Could you check a few things on this model? Use its own coordinates, in mm. Face numbers are marked on the shaded views. A direction names the side the tool comes from. Coordinates: 2 decimals unless noted, no trailing zeros. Loops run counter-clockwise (first coordinate to the right, second up) from the corner with the lowest first, then second, coordinate; pieces in that order, holes last. Notation, with made-up numbers: M 13,-21.75 L 52,-21.75 A17 cw 52,4.25 Z; hole C -32,65.5 d9. An arc over 180 degrees is marked long. Write each question's results on one line, items separated by ' | '.
```python
from build123d import *

# Parameters (mm, degrees)
BOSS_EXTRUDE1_DEPTH               = 25.4
BOSS_EXTRUDE1_DEPTH_BACK          = 25.4
SKETCH1_R                         = 4.445
SKETCH9_W                         = 30.48
SKETCH9_H                         = 35.052
CUT_EXTRUDE6_DEPTH                = 75.08914513
BOSS_EXTRUDE3_DEPTH               = 12.7
SKETCH11_W                        = 5.350768363
SKETCH11_H                        = 57.15
CUT_EXTRUDE7_DEPTH                = 94.35417198
SKETCH12_W                        = 30.48
SKETCH12_H                        = 19.05
CUT_EXTRUDE8_DEPTH                = 93.670395825
SKETCH14_R                        = 1.6
CUT_EXTRUDE9_DEPTH                = 81.005571081
SKETCH15_R                        = 3.429
CUT_EXTRUDE10_DEPTH               = 81.005571081
CUT_EXTRUDE11_DEPTH               = 2.778125
SKETCH22_W                        = 1.89865
SKETCH22_H                        = 38.369875
SKETCH23_R                        = 3.175
CUT_EXTRUDE12_DEPTH               = 22.225
SKETCH24_W                        = 43.18
SKETCH24_H                        = 41.402
CUT_EXTRUDE13_DEPTH               = 94.35417198
CUT_EXTRUDE14_REACH               = 74.389
SKETCH25_W                        = 12.7
SKETCH25_H                        = 19.05
CUT_EXTRUDE15_DEPTH               = 74.112136493
CUT_EXTRUDE15_DEPTH_BACK          = 74.112136493
SKETCH26_W                        = 19.05
SKETCH26_H                        = 61.020370042
F_25_0_1495_DIAMETER_HOLE1_REACH  = 58.443
F_25_0_1495_DIAMETER_HOLE1_BORE_R = 1.89865


with BuildPart() as part:
    # Sketch1 → Boss-Extrude1 (new, two sides: drawn at the far end of the back side and taken through both)
    with BuildSketch(Plane.XY.offset(-BOSS_EXTRUDE1_DEPTH_BACK)):
        with BuildLine():
            Line((-26.940768363, -17.415768363), (-26.940768363, 39.734231637))
            Line((-26.940768363, 39.734231637), (26.940768363, 39.734231637))
            Line((26.940768363, 39.734231637), (26.940768363, -17.415768363))
            ThreePointArc((26.940768363, -17.415768363), (36.465768363, -26.940768363), (26.940768363, -36.465768363))
            Line((26.940768363, -36.465768363), (-26.940768363, -36.465768363))
            ThreePointArc((-26.940768363, -36.465768363), (-36.465768363, -26.940768363), (-26.940768363, -17.415768363))
        make_face()
        with Locations((-26.940768363, -26.940768363)):
            Circle(SKETCH1_R, mode=Mode.SUBTRACT)
        with Locations((26.940768363, -26.940768363)):
            Circle(SKETCH1_R, mode=Mode.SUBTRACT)
    extrude(amount=BOSS_EXTRUDE1_DEPTH + BOSS_EXTRUDE1_DEPTH_BACK)

    # Sketch9 → Cut-Extrude6 (cut, through all)
    with BuildSketch(Plane.XY.offset(25.4)):
        with Locations((0, 22.208231637)):
            Rectangle(SKETCH9_W, SKETCH9_H)
    extrude(amount=-CUT_EXTRUDE6_DEPTH, mode=Mode.SUBTRACT)

    # Sketch10 → Boss-Extrude3 (add)
    with BuildSketch(Plane.XY.offset(25.4)):
        Polygon((-26.940768363, 39.734231637), (-26.940768363, -1.667768363), (26.940768363, -1.667768363), (26.940768363, 39.734231637), (15.24, 39.734231637), (15.24, 4.682231637), (-15.24, 4.682231637), (-15.24, 39.734231637), align=None)
    boss_extrude3 = extrude(amount=BOSS_EXTRUDE3_DEPTH)

    # Mirror4: Boss-Extrude3 across plane
    add(boss_extrude3.mirror(Plane.XY))

    # Sketch11 → Cut-Extrude7 (cut, through all)
    with BuildSketch(Plane.XY.offset(38.1)):
        with Locations((-24.265384181, 11.159231637)):
            Rectangle(SKETCH11_W, SKETCH11_H)
    cut_extrude7 = extrude(amount=-CUT_EXTRUDE7_DEPTH, mode=Mode.SUBTRACT)

    # Mirror5: Cut-Extrude7 across plane
    add(cut_extrude7.mirror(Plane(origin=(0, 0, 0), x_dir=(0, 0, 1), z_dir=(1, 0, 0))), mode=Mode.SUBTRACT)

    # Sketch12 → Cut-Extrude8 (cut, through all)
    with BuildSketch(Plane.XZ.offset(36.465768363)):
        Rectangle(SKETCH12_W, SKETCH12_H)
    extrude(amount=-CUT_EXTRUDE8_DEPTH, mode=Mode.SUBTRACT)

    # Sketch14 → Cut-Extrude9 (cut, through all)
    with BuildSketch(Plane.ZY.offset(21.59)):
        with Locations(Location((-18.4, 22.462231637, 0), (0, 0, 90))):
            Circle(SKETCH14_R)
    cut_extrude9 = extrude(amount=-CUT_EXTRUDE9_DEPTH, mode=Mode.SUBTRACT)

    # Mirror6: Cut-Extrude9 across plane
    add(cut_extrude9.mirror(Plane.XY), mode=Mode.SUBTRACT)

    # Sketch15 → Cut-Extrude10 (cut, through all)
    with BuildSketch(Plane(origin=(21.59, 0, 0), x_dir=(0, 0, -1), z_dir=(1, 0, 0))):
        with Locations(Location((0, 22.462231637, 0), (0, 0, 90))):
            Circle(SKETCH15_R)
    extrude(amount=-CUT_EXTRUDE10_DEPTH, mode=Mode.SUBTRACT)

    # Sketch18 → Cut-Extrude11 (cut)
    with BuildSketch(Plane(origin=(0, 4.682231637, 0), x_dir=(1, 0, 0), z_dir=(0, 1, 0))):
        Polygon((-15.24, 2.346351494), (-19.304, 4.692702988), (-23.368, 2.346351494), (-23.368, -2.346351494), (-19.304, -4.692702988), (-15.24, -2.346351494), align=None)
    cut_extrude11 = extrude(amount=-CUT_EXTRUDE11_DEPTH, mode=Mode.SUBTRACT)

    # Mirror7: Cut-Extrude11 across plane
    add(cut_extrude11.mirror(Plane(origin=(0, 0, 0), x_dir=(0, 0, 1), z_dir=(1, 0, 0))), mode=Mode.SUBTRACT)

    # Sketch22 → #6 Clearance Hole1 (revolve, cut)
    with BuildSketch(Plane(origin=(0, 1.904106637, -19.05), x_dir=(0, 0, 1), z_dir=(1, 0, 0))):
        with Locations((0.949325, 19.1849375)):
            Rectangle(SKETCH22_W, SKETCH22_H)
    f_6_clearance_hole1 = revolve(axis=Axis((0, 8.254106637, -19.05), (0, -1, 0)), mode=Mode.SUBTRACT)

    # Mirror8: #6 Clearance Hole1 across plane
    add(f_6_clearance_hole1.mirror(Plane.XY), mode=Mode.SUBTRACT)

    # Sketch23 → Cut-Extrude12 (cut)
    with BuildSketch(Plane.XZ.offset(36.465768363)):
        with Locations(Location((0, -19.05, 0), (0, 0, 270))):
            Circle(SKETCH23_R)
        with Locations(Location((0, 19.05, 0), (0, 0, 270))):
            Circle(SKETCH23_R)
    extrude(amount=-CUT_EXTRUDE12_DEPTH, mode=Mode.SUBTRACT)

    # Sketch24 → Cut-Extrude13 (cut, through all)
    with BuildSketch(Plane(origin=(0, 0, -38.1), x_dir=(-1, 0, 0), z_dir=(0, 0, -1))):
        with Locations((0, 19.033231637)):
            Rectangle(SKETCH24_W, SKETCH24_H)
    extrude(amount=-CUT_EXTRUDE13_DEPTH, mode=Mode.SUBTRACT)

    # Sketch25 → Cut-Extrude14 (cut, up to next)
    with BuildSketch(Plane.XY.offset(25.4), mode=Mode.PRIVATE) as cut_extrude14_sk1:
        with Locations((0, -19.05)):
            Rectangle(SKETCH25_W, SKETCH25_H)
    cut_extrude14_tool1 = extrude(cut_extrude14_sk1.sketch, amount=-CUT_EXTRUDE14_REACH, mode=Mode.PRIVATE) & part.part
    add(cut_extrude14_tool1.solids().sort_by_distance((0, -19.05, 25.4))[0], mode=Mode.SUBTRACT)

    # Sketch26 → Cut-Extrude15 (cut, two sides: drawn at the far end of the back side and taken through both)
    with BuildSketch(Plane(origin=(21.59, 0, 0), x_dir=(0, 0, -1), z_dir=(1, 0, 0)).offset(-CUT_EXTRUDE15_DEPTH_BACK)):
        with Locations((0, -47.925953384)):
            Rectangle(SKETCH26_W, SKETCH26_H)
    extrude(amount=CUT_EXTRUDE15_DEPTH + CUT_EXTRUDE15_DEPTH_BACK, mode=Mode.SUBTRACT)

    # #25 (0.1495) Diameter Hole1 bore → #25 (0.1495) Diameter Hole1 (cut, up to next)
    with BuildSketch(Plane(origin=(0, -36.465768363, 0), x_dir=(-1, 0, 0), z_dir=(0, -1, 0)), mode=Mode.PRIVATE) as f_25_0_1495_diameter_hole1_sk1:
        with Locations((26.940768363, -17.4625)):
            Circle(F_25_0_1495_DIAMETER_HOLE1_BORE_R)
    f_25_0_1495_diameter_hole1_tool1 = extrude(f_25_0_1495_diameter_hole1_sk1.sketch, amount=-F_25_0_1495_DIAMETER_HOLE1_REACH, mode=Mode.PRIVATE) & part.part
    # #25 (0.1495) Diameter Hole1 bore → #25 (0.1495) Diameter Hole1 (cut, up to next)
    with BuildSketch(Plane(origin=(0, -36.465768363, 0), x_dir=(-1, 0, 0), z_dir=(0, -1, 0)), mode=Mode.PRIVATE) as f_25_0_1495_diameter_hole1_sk2:
        with Locations((26.940768363, 17.4625)):
            Circle(F_25_0_1495_DIAMETER_HOLE1_BORE_R)
    f_25_0_1495_diameter_hole1_tool2 = extrude(f_25_0_1495_diameter_hole1_sk2.sketch, amount=-F_25_0_1495_DIAMETER_HOLE1_REACH, mode=Mode.PRIVATE) & part.part
    # #25 (0.1495) Diameter Hole1 bore → #25 (0.1495) Diameter Hole1 (cut, up to next)
    with BuildSketch(Plane(origin=(0, -36.465768363, 0), x_dir=(-1, 0, 0), z_dir=(0, -1, 0)), mode=Mode.PRIVATE) as f_25_0_1495_diameter_hole1_sk3:
        with Locations((-26.940768363, 17.4625)):
            Circle(F_25_0_1495_DIAMETER_HOLE1_BORE_R)
    f_25_0_1495_diameter_hole1_tool3 = extrude(f_25_0_1495_diameter_hole1_sk3.sketch, amount=-F_25_0_1495_DIAMETER_HOLE1_REACH, mode=Mode.PRIVATE) & part.part
    # #25 (0.1495) Diameter Hole1 bore → #25 (0.1495) Diameter Hole1 (cut, up to next)
    with BuildSketch(Plane(origin=(0, -36.465768363, 0), x_dir=(-1, 0, 0), z_dir=(0, -1, 0)), mode=Mode.PRIVATE) as f_25_0_1495_diameter_hole1_sk4:
        with Locations((-26.940768363, -17.4625)):
            Circle(F_25_0_1495_DIAMETER_HOLE1_BORE_R)
    f_25_0_1495_diameter_hole1_tool4 = extrude(f_25_0_1495_diameter_hole1_sk4.sketch, amount=-F_25_0_1495_DIAMETER_HOLE1_REACH, mode=Mode.PRIVATE) & part.part
    add(f_25_0_1495_diameter_hole1_tool1.solids().sort_by_distance((-26.940768, -36.465768, 17.4625))[0], mode=Mode.SUBTRACT)
    add(f_25_0_1495_diameter_hole1_tool2.solids().sort_by_distance((-26.940768, -36.465768, -17.4625))[0], mode=Mode.SUBTRACT)
    add(f_25_0_1495_diameter_hole1_tool3.solids().sort_by_distance((26.940768, -36.465768, -17.4625))[0], mode=Mode.SUBTRACT)
    add(f_25_0_1495_diameter_hole1_tool4.solids().sort_by_distance((26.940768, -36.465768, 17.4625))[0], mode=Mode.SUBTRACT)


solid = part.part
```
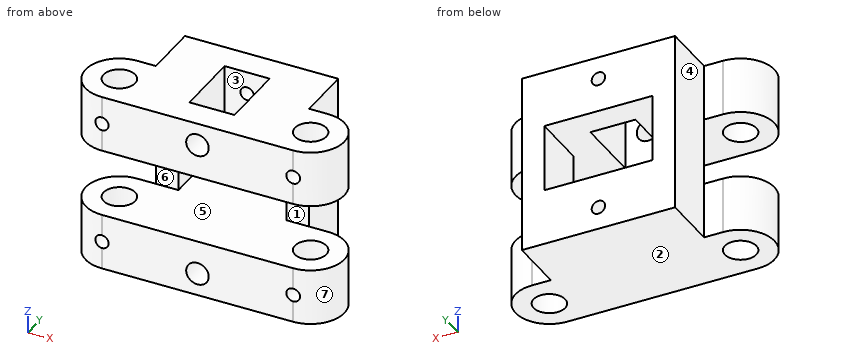
(1) Imagine slicing it at D-D, the plane z = 11. List the corners of the cut face in (x, y) for me (3 decimals).
Reported:
outline: M -26.941,-36.466 L 26.941,-36.466 A9.525 ccw 26.941,-17.416 L 21.59,-17.416 L 21.59,-1.668 L -21.59,-1.668 L -21.59,-17.416 L -26.941,-17.416 A9.525 ccw Z; hole C -26.941,-26.941 d8.89; hole M -6.35,-28.575 L 6.35,-28.575 L 6.35,-9.525 L -6.35,-9.525 Z; hole C 26.941,-26.941 d8.89
(2) Imagine slicing it at C-C, the plane y = -10.5. List the corners of the cut face in (x, z) for me (3 decimals), and give its area (3 significant figures).
Reported:
outline: M -21.59,-25.4 L 21.59,-25.4 L 21.59,25.4 L 6.35,25.4 L 6.35,9.525 L 15.24,9.525 L 15.24,-9.525 L -15.24,-9.525 L -15.24,9.525 L -6.35,9.525 L -6.35,25.4 L -21.59,25.4 Z; hole C 0,-19.05 d3.797 | area: 1,400 mm2
(3) Please list where these lines run through material, in increasing order: probe 1 along X at (y, z) = (-7.5, 19.05); probe 2 along X at (y, z) = (-11, 23.5); probe 3 along X at (y, z) = (-24.5, 21.5). Write a range as from..to.
Reported:
probe 1: x = -21.59..-1.9, 1.9..21.59 | probe 2: x = -21.59..-6.35, 6.35..21.59 | probe 3: x = -36.15..-30.66, -23.23..-6.35, 6.35..23.23, 30.66..36.15
(4) If we mould it in two halves opening along Y, with no side actions, what happens to the marked faces 1, 2 and 3? For each: released by +Y, released by -Y, zero draft, split by the parting line, or undercut.
Reported:
face 1: released by -Y | face 2: zero draft | face 3: undercut
(5) Imagine slicing it at B-B, the plane x = 0. List the corners of the cut face in (y, z) for me (3 decimals).
Reported:
outline: M -36.466,-25.4 L -1.668,-25.4 L -1.668,-20.949 L -14.241,-20.949 L -14.241,-22.225 L -36.466,-22.225 Z; M -36.466,-15.875 L -14.241,-15.875 L -14.241,-17.151 L -1.668,-17.151 L -1.668,-9.525 L -36.466,-9.525 Z; M -36.466,9.525 L -28.575,9.525 L -28.575,15.875 L -36.466,15.875 Z; M -36.466,22.225 L -28.575,22.225 L -28.575,25.4 L -36.466,25.4 Z; M -9.525,9.525 L -1.668,9.525 L -1.668,17.151 L -9.525,17.151 Z; M -9.525,20.949 L -1.668,20.949 L -1.668,25.4 L -9.525,25.4 Z
(6) Which directions (+Z, -Z, +X, -X, +Y, -Y) give clear straight access to the entire face, cutting with the end or side of a thin tool? Please do the marked faces 4, 5, 6 and 7.
Reported:
face 4: +Z, -Z, -X, +Y | face 5: -Y | face 6: +X, -X, -Y | face 7: +Z, -Z, +X
(7) Imagine slicing it at A-A, the plane y = -5.5. List the corners of the cut face in (x, z) for me (3 decimals), and give its area (3 significant figures).
Reported:
outline: M -21.59,-25.4 L 21.59,-25.4 L 21.59,25.4 L -21.59,25.4 Z; hole M -15.24,-9.525 L 15.24,-9.525 L 15.24,9.525 L -15.24,9.525 Z; hole C 0,-19.05 d3.797; hole C 0,19.05 d3.797 | area: 1,590 mm2
(8) Will these pins go through, and if not, where does the flat tip stop? P1, Ø8, axis at x = 4, z = 2, coming from the +Y side; P2, Ø12.5, axis at y = -13, z = 3, coming from the -X side; P3, Ø5, axis at y = -21, z = 20, coming from the +X side; P4, Ø4.5, axis at y = -12, z = -4.5, coming from the +X side.
Reported:
P1: passes through | P2: stops at x = -21.59 | P3: stops at x = 35.82 | P4: stops at x = 21.59
